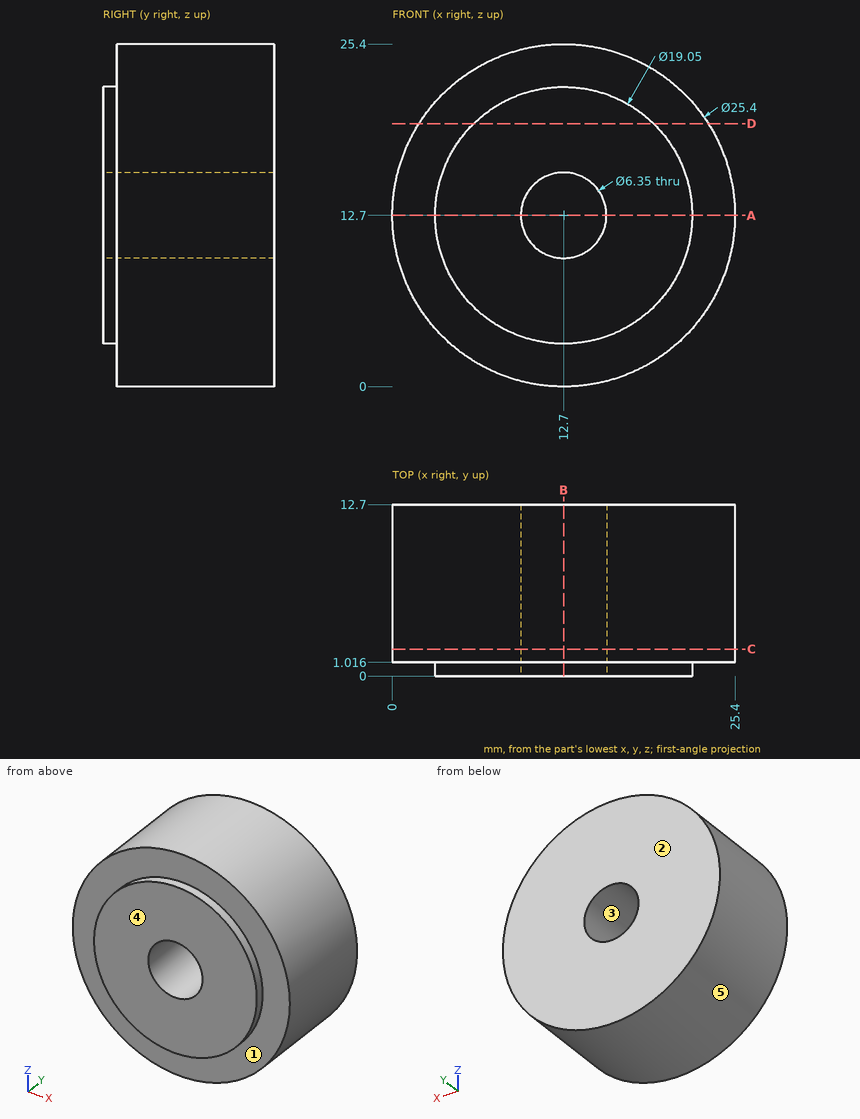
For this review, use the dimensioned drawing (mm, ordinates from the lowest corner) and the shaded views. A direction names the side the tool comes from. Coordinates: 2 decimals unless noted, no trailing zeros. Loops run counter-clockwise (first coordinate to the right, second up) from the corner with the lowest first, then second, coordinate; pieces in that order, holes last. Notation, with made-up numbers: (3, -33) - (17, -33) arc R18 ccw to (17, -5) - close; hole circle Ø6 at (37.25, 66). An arc over 180 degrees is marked (long way). Use one line per item in the form item = value. Start each with the question number.
1) For the marked faces 1 and 2, list the 3-axis set-ups (+Z, -Z, +X, -X, +Y, -Y) from which the entire face can be reached by the end or side of a thin tool; tool diameter is ignored.
2) Take a section at B-B (x = 12.7). State the section outline as (y, z) points (3 decimals), plus the area to 3 significant figures.
3) To check wall thickness, follow probe 1 along Z at (x, y) = (12.7, 5.75) (3 decimals); probe 2 along Y at (x, z) = (7.5, 22.5). State the ranges of each line that lie inside material, in increasing order. Write a range as from..to.
4) Draft analysis for pull direction Z (two halves, no side actions). For the marked faces 3, 4 and 5, state which applies: released by +Z, released by -Z, zero draft, split by the parting line, or undercut.
5) For pin 1 (6 mm diameter, centred on x = 18, y = 8, fed in from +Z); pin 2 (2 mm diameter, centred on x = 12.5, z = 13.5, fed in from +Y); pin 3 (2 mm diameter, centred on y = 3.5, z = 6.5, fed in from -X); pin 4 (4 mm diameter, centred on x = 5.5, y = 10.5, fed in from +Z), all flat-tipped, find the tip position at first contact; note any pin that passes through.
6) Take a section at C-C (y = 2). State the section outline as (x, z) points (3 decimals).
7) Take a section at A-A (z = 12.7). State the section outline as (x, y) points (3 decimals), plus the area to 3 significant figures.
8) Take a section at D-D (z = 19.5). State the section outline as (x, y) points, plus the area to 3 significant figures.
From the geometry:
q1.face_1 = -Y
q1.face_2 = +Z, -Z, +X, -X, +Y
q2.outline = (0, 3.175) - (1.016, 3.175) - (1.016, 0) - (12.7, 0) - (12.7, 9.525) - (0, 9.525) - close; (0, 15.875) - (12.7, 15.875) - (12.7, 25.4) - (1.016, 25.4) - (1.016, 22.225) - (0, 22.225) - close
q2.area = 235 mm2
q3.probe_1 = 0..9.525, 15.875..25.4
q3.probe_2 = 1.02..12.7
q4.face_3 = undercut
q4.face_4 = zero draft
q4.face_5 = split by the parting line
q5.pin_1 = 25.19
q5.pin_2 = through
q5.pin_3 = 1.11
q5.pin_4 = 24.29
q6.outline = circle Ø25.4 at (12.7, 12.7); hole circle Ø6.35 at (12.7, 12.7)
q7.outline = (0, 1.016) - (3.175, 1.016) - (3.175, 0) - (9.525, 0) - (9.525, 12.7) - (0, 12.7) - close; (15.875, 0) - (22.225, 0) - (22.225, 1.016) - (25.4, 1.016) - (25.4, 12.7) - (15.875, 12.7) - close
q7.area = 235 mm2
q8.outline = (1.97, 1.02) - (6.03, 1.02) - (6.03, 0) - (19.37, 0) - (19.37, 1.02) - (23.43, 1.02) - (23.43, 12.7) - (1.97, 12.7) - close
q8.area = 264 mm2
